from build123d import *
from build123d.topology import SkipClean

# Parameters (mm, degrees)
SKETCH1_R                            = 30
BOSS_EXTRUDE1_DEPTH                  = 4
BOSS_EXTRUDE2_REACH                  = 44.615
BOSS_EXTRUDE2_END_RADIUS             = 30
BOSS_EXTRUDE2_DIRECTION_2_REACH      = 44.615
BOSS_EXTRUDE2_DIRECTION_2_END_RADIUS = 30
SKETCH3_OUTSIDE_W                    = 78.092
SKETCH3_OUTSIDE_H                    = 69.092
SKETCH3_OUTSIDE_R                    = 21.5
CUT_EXTRUDE2_DEPTH                   = 12.5
BOSS_EXTRUDE3_DEPTH                  = 18
BOSS_EXTRUDE4_DEPTH                  = 15
BOSS_EXTRUDE5_DEPTH                  = 15
CUT_EXTRUDE3_DEPTH                   = 44.292609069
CUT_EXTRUDE3_DEPTH_BACK              = 44.292609069
SKETCH8_R                            = 2
CUT_EXTRUDE8_DEPTH                   = 48.077064479
CUT_EXTRUDE8_DEPTH_BACK              = 48.077064479
CUT_EXTRUDE9_DEPTH                   = 59.659818207
CUT_EXTRUDE11_DEPTH                  = 20
CUT_EXTRUDE12_DEPTH                  = 20
CUT_EXTRUDE13_DEPTH                  = 20
CUT_EXTRUDE14_DEPTH                  = 44.292609069
CUT_EXTRUDE14_DEPTH_BACK             = 44.292609069
SKETCH25_W                           = 66.075437062
SKETCH25_H                           = 20.142243048
SKETCH26_R                           = 5
CUT_EXTRUDE15_DEPTH                  = 24
SKETCH27_R                           = 1.5
CUT_EXTRUDE16_DEPTH                  = 30
SKETCH28_R                           = 5
CUT_EXTRUDE17_DEPTH                  = 3


with BuildPart() as part:
    # Sketch1 → Boss-Extrude1 (new body)
    with BuildSketch(Plane(origin=(0, 0, 0), x_dir=(1, 0, 0), z_dir=(0, 1, 0))):
        with Locations(Location((0, 0, 0), (0, 0, 270))):
            Circle(SKETCH1_R)
    extrude(amount=BOSS_EXTRUDE1_DEPTH)

    # Boss-Extrude2: up to this cylinder (the profile starts inside it)
    with SkipClean():  # the faces are left unmerged after this step: merging them gives an invalid solid
        boss_extrude2_end = Plane(origin=(0, 9.396175, 0), z_dir=(0, -1, 0)) * Cylinder(BOSS_EXTRUDE2_END_RADIUS, 150.23, mode=Mode.PRIVATE)
        # Sketch2 → Boss-Extrude2 (add, up to the surface)
        with BuildSketch(Plane(origin=(0, 0, 0), x_dir=(0, 0, -1), z_dir=(1, 0, 0)), mode=Mode.PRIVATE) as boss_extrude2_sk1:
            Polygon((0, 4), (21.5, 4), (9, 16.5), (-9, 16.5), (-21.5, 4), align=None)
        boss_extrude2_tool1 = extrude(boss_extrude2_sk1.sketch, amount=BOSS_EXTRUDE2_REACH, mode=Mode.PRIVATE) & boss_extrude2_end
        add(boss_extrude2_tool1.solids().sort_by_distance((0, 9.396175, 0))[0])

    # Boss-Extrude2 direction 2: up to this cylinder (the profile starts inside it)
    with SkipClean():  # the faces are left unmerged after this step: merging them gives an invalid solid
        boss_extrude2_direction_2_end = Plane(origin=(0, 9.396175, 0), z_dir=(0, -1, 0)) * Cylinder(BOSS_EXTRUDE2_DIRECTION_2_END_RADIUS, 150.23, mode=Mode.PRIVATE)
        # Sketch2 → Boss-Extrude2 direction 2 (add, up to the surface)
        with BuildSketch(Plane(origin=(0, 0, 0), x_dir=(0, 0, -1), z_dir=(1, 0, 0)), mode=Mode.PRIVATE) as boss_extrude2_direction_2_sk1:
            Polygon((0, 4), (21.5, 4), (9, 16.5), (-9, 16.5), (-21.5, 4), align=None)
        boss_extrude2_direction_2_tool1 = extrude(boss_extrude2_direction_2_sk1.sketch, amount=-BOSS_EXTRUDE2_DIRECTION_2_REACH, mode=Mode.PRIVATE) & boss_extrude2_direction_2_end
        add(boss_extrude2_direction_2_tool1.solids().sort_by_distance((0, 9.396175, 0))[0])

    # SurfaceCut1
    split(bisect_by=Plane(origin=(0, 12.75, -12.75), x_dir=(1, 0, 0), z_dir=(0, 0.7071067811865558, -0.7071067811865392)), keep=Keep.BOTTOM)

    # SurfaceCut2
    split(bisect_by=Plane(origin=(0, 12.75, 12.75), x_dir=(1, 0, 0), z_dir=(0, 0.7071067811865509, 0.7071067811865442)), keep=Keep.BOTTOM)

    # Sketch3 outside → Cut-Extrude2 (cut)
    with SkipClean():  # the faces are left unmerged after this step: merging them gives an invalid solid
        with BuildSketch(Plane(origin=(0, 4, 0), x_dir=(1, 0, 0), z_dir=(0, 1, 0))):
            Rectangle(SKETCH3_OUTSIDE_W, SKETCH3_OUTSIDE_H)
            Circle(SKETCH3_OUTSIDE_R, mode=Mode.SUBTRACT)
        extrude(amount=CUT_EXTRUDE2_DEPTH, mode=Mode.SUBTRACT)

    # Sketch5 → Boss-Extrude3 (add)
    with SkipClean():  # the faces are left unmerged after this step: merging them gives an invalid solid
        with BuildSketch(Plane(origin=(0, 0, 0), x_dir=(-1, 0, 0), z_dir=(0, -1, 0))):
            Polygon((0, -6), (-17.5, -6), (-17.5, 6), (17.5, 6), (17.5, -6), align=None)
        extrude(amount=BOSS_EXTRUDE3_DEPTH)

    # Sketch6 → Boss-Extrude4 (add)
    with SkipClean():  # the faces are left unmerged after this step: merging them gives an invalid solid
        with BuildSketch(Plane.XZ):
            Polygon((0, 15), (7, 15), (7, 6), (-7, 6), (-7, 15), align=None)
        extrude(amount=BOSS_EXTRUDE4_DEPTH)

    # Sketch7 → Boss-Extrude5 (add)
    with SkipClean():  # the faces are left unmerged after this step: merging them gives an invalid solid
        with BuildSketch(Plane.XZ):
            Polygon((0, -15), (7, -15), (7, -6), (-7, -6), (-7, -15), align=None)
        extrude(amount=BOSS_EXTRUDE5_DEPTH)

    # Sketch8 → Cut-Extrude3 (cut, two sides: drawn at the far end of the back side and taken through both)
    with SkipClean():  # the faces are left unmerged after this step: merging them gives an invalid solid
        with BuildSketch(Plane.XY.offset(-CUT_EXTRUDE3_DEPTH_BACK)):
            with Locations((-12.5, -12.5)):
                Circle(SKETCH8_R)
            with Locations((12.5, -12.5)):
                Circle(SKETCH8_R)
        extrude(amount=CUT_EXTRUDE3_DEPTH + CUT_EXTRUDE3_DEPTH_BACK, mode=Mode.SUBTRACT)

    # Sketch16 → Cut-Extrude8 (cut, two sides: drawn at the far end of the back side and taken through both)
    with SkipClean():  # the faces are left unmerged after this step: merging them gives an invalid solid
        with BuildSketch(Plane.XY.offset(6).offset(-CUT_EXTRUDE8_DEPTH_BACK)):
            Polygon((17.5, -18), (17.5, -14.5), (14, -18), align=None)
            Polygon((-17.5, -18), (-14, -18), (-17.5, -14.5), align=None)
        extrude(amount=CUT_EXTRUDE8_DEPTH + CUT_EXTRUDE8_DEPTH_BACK, mode=Mode.SUBTRACT)

    # Sketch17 → Cut-Extrude9 (cut, through all)
    with SkipClean():  # the faces are left unmerged after this step: merging them gives an invalid solid
        with BuildSketch(Plane(origin=(10.365975269, -9.674910251, -8.062425209), x_dir=(-0.3613483622370374, 0.337258471421235, -0.8693009171531012), z_dir=(0.6355070151731325, -0.5931398808282571, -0.49428323402354774))):
            Polygon((-2.372510104, -6.189601271), (7.980636686, -0.706686759), (7.980636686, -10.965829024), align=None)
        extrude(amount=CUT_EXTRUDE9_DEPTH, mode=Mode.SUBTRACT)

    # Sketch19 → Cut-Extrude11 (cut)
    with SkipClean():  # the faces are left unmerged after this step: merging them gives an invalid solid
        with BuildSketch(Plane(origin=(-10.365975269, -9.674910251, -8.062425209), x_dir=(0.3613483622370374, 0.33725847142123494, -0.8693009171531012), z_dir=(0.6355070151731324, 0.5931398808282571, 0.4942832340235476))):
            Polygon((-2.372510104, -6.189601271), (7.980636686, -10.965829024), (7.980636686, -0.706686759), align=None)
        extrude(amount=-CUT_EXTRUDE11_DEPTH, mode=Mode.SUBTRACT)

    # Sketch20 → Cut-Extrude12 (cut)
    with SkipClean():  # the faces are left unmerged after this step: merging them gives an invalid solid
        with BuildSketch(Plane(origin=(-10.365975269, -9.674910251, 8.062425209), x_dir=(-0.3613483622370374, -0.3372584714212349, -0.8693009171531013), z_dir=(0.6355070151731326, 0.593139880828257, -0.49428323402354757))):
            Polygon((2.372510104, -6.189601271), (-7.980636686, -0.706686759), (-7.980636686, -10.965829024), align=None)
        extrude(amount=-CUT_EXTRUDE12_DEPTH, mode=Mode.SUBTRACT)

    # Sketch21 → Cut-Extrude13 (cut)
    with SkipClean():  # the faces are left unmerged after this step: merging them gives an invalid solid
        with BuildSketch(Plane(origin=(10.365975269, -9.674910251, 8.062425209), x_dir=(-0.3613483622370374, 0.3372584714212349, 0.8693009171531013), z_dir=(-0.6355070151731326, 0.593139880828257, -0.49428323402354757))):
            Polygon((-2.372510104, -6.189601271), (7.980636686, -0.706686759), (7.980636686, -10.965829024), align=None)
        extrude(amount=-CUT_EXTRUDE13_DEPTH, mode=Mode.SUBTRACT)

    # Sketch25 → Cut-Extrude14 (cut, two sides: drawn at the far end of the back side and taken through both)
    with SkipClean():  # the faces are left unmerged after this step: merging them gives an invalid solid
        with BuildSketch(Plane.XY.offset(-CUT_EXTRUDE14_DEPTH_BACK)):
            with Locations((0, -10.071121524)):
                Rectangle(SKETCH25_W, SKETCH25_H)
        extrude(amount=CUT_EXTRUDE14_DEPTH + CUT_EXTRUDE14_DEPTH_BACK, mode=Mode.SUBTRACT)

    # Sketch26 → Cut-Extrude15 (cut)
    with SkipClean():  # the faces are left unmerged after this step: merging them gives an invalid solid
        with BuildSketch(Plane(origin=(0, 16.5, 0), x_dir=(1, 0, 0), z_dir=(0, 1, 0))):
            with Locations(Location((-8, 0, 0), (0, 0, 270))):
                Circle(SKETCH26_R)
            with Locations(Location((8, 0, 0), (0, 0, 270))):
                Circle(SKETCH26_R)
        extrude(amount=-CUT_EXTRUDE15_DEPTH, mode=Mode.SUBTRACT)

    # Sketch27 → Cut-Extrude16 (cut)
    with SkipClean():  # the faces are left unmerged after this step: merging them gives an invalid solid
        with BuildSketch(Plane(origin=(0, 16.5, 0), x_dir=(1, 0, 0), z_dir=(0, 1, 0))):
            with Locations(Location((0, 0, 0), (0, 0, 270))):
                Circle(SKETCH27_R)
        extrude(amount=-CUT_EXTRUDE16_DEPTH, mode=Mode.SUBTRACT)

    # Sketch28 → Cut-Extrude17 (cut)
    with SkipClean():  # the faces are left unmerged after this step: merging them gives an invalid solid
        with BuildSketch(Plane.XZ):
            with Locations(Location((0, -15, 0), (0, 0, 270))):
                Circle(SKETCH28_R)
            with Locations(Location((22, 0, 0), (0, 0, 270))):
                Circle(SKETCH28_R)
            with Locations(Location((0, 15, 0), (0, 0, 270))):
                Circle(SKETCH28_R)
            with Locations(Location((-22, 0, 0), (0, 0, 270))):
                Circle(SKETCH28_R)
            with Locations(Location((-14, 12, 0), (0, 0, 270))):
                Circle(SKETCH28_R)
            with Locations(Location((14, 12, 0), (0, 0, 270))):
                Circle(SKETCH28_R)
            with Locations(Location((14, -12, 0), (0, 0, 270))):
                Circle(SKETCH28_R)
            with Locations(Location((-14, -12, 0), (0, 0, 270))):
                Circle(SKETCH28_R)
        extrude(amount=-CUT_EXTRUDE17_DEPTH, mode=Mode.SUBTRACT)


solid = part.part
Source: CAD feature listing. Evaluate the final solid. Frame: model axes, mm. A direction names the side the tool comes from. Coordinates: 2 decimals unless noted, no trailing zeros. Order: outer loops, then holes, each group sorted by start corner. A loop starts at its lowest first (then second) coordinate and runs counter-clockwise, first axis right, second up. Notation, with made-up numbers: M -3,9 L 25,9 A26 cw 25,23 Z; hole C 0.5,-31.75 d3. An arc over 180 degrees is marked long. Write each question's results on one line, items separated by ' | '. Start each with the question number.
Item 1: Draft query along X for faces 1 (the face through (30, 2, 0)), 2 (the face through (-30, 2, 0)), 3 (the face through (14, 3, 12)), 4 (the face through (0.3, 11.6, -13.9)). Return one class per face: pulls with the +X half, pulls with the -X half, needs draft (parallel to the pull), parting line crosses it, or undercut.
Item 2: Cut plane A-A (y = 8). Return loops of the section in (x, z), and give its area (3 significant figures).
Item 3: Cut plane D-D (y = 1.25). Count the separate pieces of the cut face and the enclosed holes in it, and give its area (3 significant figures).
Item 4: Cut plane C-C (z = 12). Return loops of the section in (x, y), and give its area (3 significant figures).
Item 5: Set-up query: faces 5 (the face through (23, 4, -2)), 6 (the face through (22, 3, 0)), 7 (the face through (0.3, 11.7, 13.8)). Return all of +Z, -Z, +X, -X, +Y, -Y with unobstructed straight access to the full face (end or side cutting, diameter ignored); none if empty.
Item 6: Cut plane B-B (x = 8). Return loops of the section in (y, z).
Item 7: Line query: probe 1 along X at (y, z) = (7.25, 0); probe 2 along X at (y, z) = (2.15, 0); probe 3 along X at (y, z) = (11.25, 4.5). Output: solid intervals per line, ascending.
Item 8: First-contact query: pin 1 Ø6 at (x, y) = (-9.5, 13.5) entering from -Z; pin 2 Ø1.5 at (x, y) = (14.5, 12) entering from -Z; pin 3 Ø3 at (x, z) = (13.5, -12.5) entering from -Y. Flat tips, straight axial feed; report the tip coordinate or a pass-through.
Checked values:
1) face 1: pulls with the +X half | face 2: pulls with the -X half | face 3: undercut | face 4: needs draft
2) outline: M -12.49,-17.5 L 12.49,-17.5 A21.5 ccw 12.49,17.5 L -12.49,17.5 A21.5 ccw Z; hole C -8,0 d10; hole C 0,0 d3; hole C 8,0 d10 | area: 1,150 mm2
3) separate pieces: 1 | enclosed holes: 11 | area: 1,760 mm2
4) outline: M -27.5,0 L -19,0 L -19,3 L -9,3 L -9,0 L -4,0 L -4,3 L 4,3 L 4,0 L 9,0 L 9,3 L 19,3 L 19,0 L 27.5,0 L 27.5,4 L 17.84,4 L 17.84,13.5 L -17.84,13.5 L -17.84,4 L -27.5,4 Z | area: 475 mm2
5) face 5: +X, +Y | face 6: -Y | face 7: +Z, +X, -X, +Y
6) outline: M 0,-25.5 L 4,-21.5 L 4,-19.96 L 5.54,-19.96 L 16.5,-9 L 16.5,-5 L 0,-5 Z; M 0,5 L 16.5,5 L 16.5,9 L 5.54,19.96 L 4,19.96 L 4,21.5 L 0,25.5 Z
7) probe 1: x = -21.5 to -13, -3 to -1.5, 1.5 to 3, 13 to 21.5 | probe 2: x = -30 to -27, -17 to -13, -3 to -1.5, 1.5 to 3, 13 to 17, 27 to 30 | probe 3: x = -21.02 to -10.18, -5.82 to 5.82, 10.18 to 21.02
8) pin 1: stops at z = -15 | pin 2: stops at z = -14.25 | pin 3: stops at y = 3
